Geometry check sheet. Reference: the model listing, model coordinates, mm. Face numbers are marked on the shaded views. Round coordinates to 2 decimals unless told otherwise and drop trailing zeros. Write each loop counter-clockwise with the first axis right and the second up, starting at its lowest first coordinate (ties: lowest second). Pieces come first, ordered by that corner, then holes.
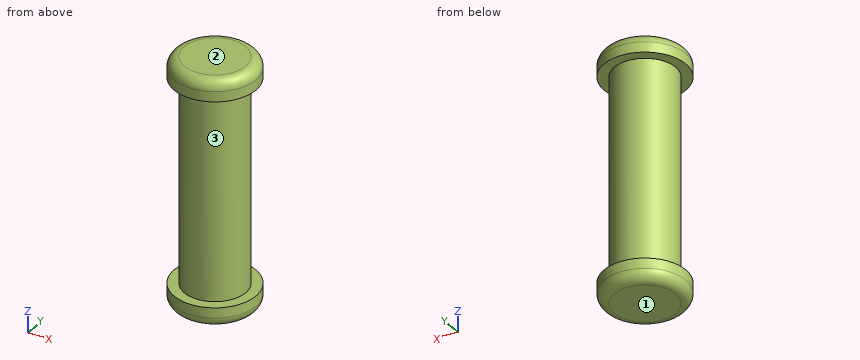
from build123d import *

# Parameters (mm, degrees)
SKETCH1_R           = 1.5
BOSS_EXTRUDE1_DEPTH = 10
SKETCH2_R           = 2
BOSS_EXTRUDE2_DEPTH = 1
SKETCH3_R           = 2
BOSS_EXTRUDE3_DEPTH = 1
FILLET1_R           = 0.5


with BuildPart() as part:
    # Sketch1 → Boss-Extrude1 (new body)
    with BuildSketch(Plane.XY):
        Circle(SKETCH1_R)
    extrude(amount=BOSS_EXTRUDE1_DEPTH)

    # Sketch2 → Boss-Extrude2 (add)
    with BuildSketch(Plane(origin=(0, 0, 0), x_dir=(-1, 0, 0), z_dir=(0, 0, -1))):
        Circle(SKETCH2_R)
    extrude(amount=BOSS_EXTRUDE2_DEPTH)

    # Sketch3 → Boss-Extrude3 (add)
    with BuildSketch(Plane.XY.offset(10)):
        Circle(SKETCH3_R)
    extrude(amount=BOSS_EXTRUDE3_DEPTH)

    # Fillet1
    fillet1_edges = [part.edges().sort_by_distance(p)[0] for p in [
        (-2, 0, 11),
        (2, 0, -1),
    ]]
    fillet(fillet1_edges, radius=FILLET1_R)


solid = part.part
1. Section check A-A (x = 0). Record the cut outline in (y, z).
2. Release check for a two-part mould opening along Z. For the marked faces 1, 2 and 3 record: +Z half, -Z half, draft (parallel to the pull), parting line (faces both ways), or undercut.
3. Scan lines: line 1 along Z through (x, y) = (0.3, -1.5); line 2 along Z through (x, y) = (1.7, -0.6); line 3 along X through (y, z) = (-1.3, -0.5). Record each from-to range of solid material in increasing order.
4. Section check C-C (z = 7.25). Record the cut outline in (x, y).
5. Depth check by flat-ended pin: pin 1 Ø1 at (y, z) = (-1, 3.5) entering from -X; pin 2 Ø1.5 at (y, z) = (-1.5, 2) entering from -X. Enter the tip coordinate at first touch or a pass-through.
Results below:
1. outline: (-2, -0.5) arc R0.5 ccw to (-1.5, -1) - (1.5, -1) arc R0.5 ccw to (2, -0.5) - (2, 0) - (1.5, 0) - (1.5, 10) - (2, 10) - (2, 10.5) arc R0.5 ccw to (1.5, 11) - (-1.5, 11) arc R0.5 ccw to (-2, 10.5) - (-2, 10) - (-1.5, 10) - (-1.5, 0) - (-2, 0) - close
2. face 1: -Z half
2. face 2: +Z half
2. face 3: undercut
3. line 1: z = -1 to 0, 10 to 11
3. line 2: z = -0.9 to 0, 10 to 10.9
3. line 3: x = -1.52 to 1.52
4. outline: circle Ø3 at (0, 0)
5. pin 1: stops at x = -1.41
5. pin 2: stops at x = -1.3
